```python
from build123d import *

# Parameters (mm, degrees)
SKETCH1_R           = 5
BOSS_EXTRUDE1_DEPTH = 20


with BuildPart() as part:
    # Sketch1 → Boss-Extrude1 (new body)
    with BuildSketch(Plane(origin=(0, 0, 0), x_dir=(1, 0, 0), z_dir=(0, 1, 0))):
        with BuildLine():
            Line((29.481516636, 13.522108771), (31.799144094, 6.389184898))
            Line((31.799144094, 6.389184898), (24.666220221, 4.071557441))
            ThreePointArc((24.666220221, 4.071557441), (23.776412907, -7.725424859), (17.562189929, -17.792399639))
            Line((17.562189929, -17.792399639), (21.970579321, -23.860027097))
            Line((21.970579321, -23.860027097), (15.902951863, -28.268416489))
            Line((15.902951863, -28.268416489), (11.494562471, -22.200789031))
            ThreePointArc((11.494562471, -22.200789031), (0, -25), (-11.494562471, -22.200789031))
            Line((-11.494562471, -22.200789031), (-15.902951863, -28.268416489))
            Line((-15.902951863, -28.268416489), (-21.970579321, -23.860027097))
            Line((-21.970579321, -23.860027097), (-17.562189929, -17.792399639))
            ThreePointArc((-17.562189929, -17.792399639), (-23.776412907, -7.725424859), (-24.666220221, 4.071557441))
            Line((-24.666220221, 4.071557441), (-31.799144094, 6.389184898))
            Line((-31.799144094, 6.389184898), (-29.481516636, 13.522108771))
            Line((-29.481516636, 13.522108771), (-22.348592764, 11.204481313))
            ThreePointArc((-22.348592764, 11.204481313), (-14.694631307, 20.225424859), (-3.75, 24.717149917))
            Line((-3.75, 24.717149917), (-3.75, 32.217149917))
            Line((-3.75, 32.217149917), (3.75, 32.217149917))
            Line((3.75, 32.217149917), (3.75, 24.717149917))
            ThreePointArc((3.75, 24.717149917), (14.694631307, 20.225424859), (22.348592764, 11.204481313))
            Line((22.348592764, 11.204481313), (29.481516636, 13.522108771))
        make_face()
        with Locations(Location((0, 0, 0), (0, 0, 270))):
            Circle(SKETCH1_R, mode=Mode.SUBTRACT)
    extrude(amount=BOSS_EXTRUDE1_DEPTH)


solid = part.part
```
Input: part model. Units: mm. Frame: model coordinates. A direction names the side the tool comes from. Coordinates: 2 decimals unless noted, no trailing zeros. Write each loop counter-clockwise with the first axis right and the second up, starting at its lowest first coordinate (ties: lowest second). Pieces come first, ordered by that corner, then holes.
1) Pin query (flat end, axial travel): pin 1 Ø10 at (y, z) = (3.5, -1.5) entering from -X; pin 2 Ø2 at (x, z) = (10, 7) entering from -Y; pin 3 Ø1 at (y, z) = (10.5, -1) entering from -X (3 decimals); pin 4 Ø4 at (y, z) = (7.5, -11.5) entering from +X. Return the tip coordinate at first contact, or that it passes through.
2) Section C-C on z = 0. Output: boundary loops of the cut face in (x, y), and give its area (3 significant figures).
3) Mould query, pull axis X, two halves, no side actions, for faces 1 (the flat face through (-7, 0, -2)), 2 (the flat face through (3.75, 10, -29)), 3 (the flat face through (-13.668, 9.86, 25.192)), 4 (the cylindrical face through (0, 10, 25)). Classes: pulls with the +X half, pulls with the -X half, needs draft (parallel to the pull), parting line crosses it, or undercut.
4) Material intervals for line 1 along X through (y, z) = (15.5, 0); line 2 along X through (y, z) = (10.5, -25); line 3 along Z through (x, y) = (-2, 18.25), sorted ascending.
5) Section D-D on z = -12. Output: boundary loops of the cut face in (x, y), and give its area (3 significant figures).
6) Set-up query: faces 5 (the flat face through (13.73, 9.86, 25.28)), 6 (the flat face through (-3.75, 10, -28)), 7 (the flat face through (-25.96, 9.86, -12.38)), 8 (the flat face through (-19.8, 9.86, 20.87)), 9 (the flat face through (19.736, 9.86, 20.784)). Return all of +Z, -Z, +X, -X, +Y, -Y with unobstructed straight access to the full face (end or side cutting, diameter ignored); none if empty.
7) Section A-A on x = 0. Output: boundary loops of the cut face in (y, z).
8) Section B-B on y = 1.5. Output: boundary loops of the cut face in (x, z).
Check result:
1. pin 1: stops at x = -31.8
1. pin 2: stops at y = 0
1. pin 3: stops at x = -24.995
1. pin 4: stops at x = 30.79
2. outline: (-25, 0) - (-5, 0) - (-5, 20) - (-25, 20) - close; (5, 0) - (25, 0) - (25, 20) - (5, 20) - close
2. area: 800 mm2
3. face 1: needs draft
3. face 2: pulls with the +X half
3. face 3: undercut
3. face 4: undercut
4. line 1: x = -25 to -5, 5 to 25
4. line 2: x = -3.75 to 3.75
4. line 3: z = -32.22 to -4.58, 4.58 to 24.92
5. outline: (-29.98, 0) - (-24.8, 0) - (-24.8, 20) - (-29.98, 20) - close; (-21.93, 0) - (21.93, 0) - (21.93, 20) - (-21.93, 20) - close; (24.8, 0) - (29.98, 0) - (29.98, 20) - (24.8, 20) - close
5. area: 1,080 mm2
6. face 5: +Z, +Y, -Y
6. face 6: -Z, -X, +Y, -Y
6. face 7: -Z, +Y, -Y
6. face 8: -X, +Y, -Y
6. face 9: +X, +Y, -Y
7. outline: (0, -32.22) - (20, -32.22) - (20, -5) - (0, -5) - close; (0, 5) - (20, 5) - (20, 25) - (0, 25) - close
8. outline: (-31.8, -6.39) - (-29.48, -13.52) - (-22.35, -11.2) arc R25 ccw to (-3.75, -24.72) - (-3.75, -32.22) - (3.75, -32.22) - (3.75, -24.72) arc R25 ccw to (22.35, -11.2) - (29.48, -13.52) - (31.8, -6.39) - (24.67, -4.07) arc R25 ccw to (17.56, 17.79) - (21.97, 23.86) - (15.9, 28.27) - (11.49, 22.2) arc R25 ccw to (-11.49, 22.2) - (-15.9, 28.27) - (-21.97, 23.86) - (-17.56, 17.79) arc R25 ccw to (-24.67, -4.07) - close; hole circle Ø10 at (0, 0)
